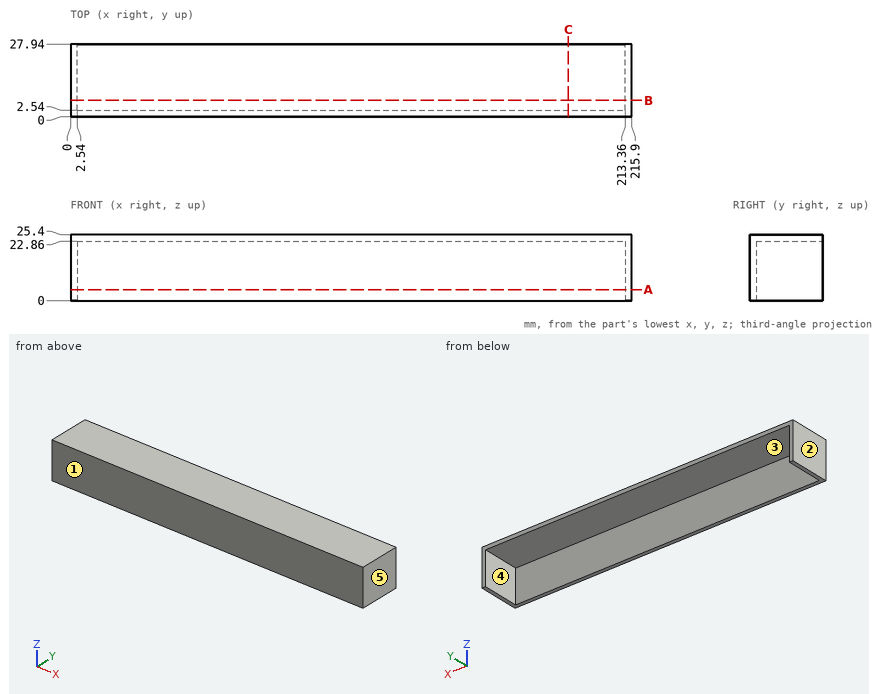
Drawing for the job (mm, zero at the part's lowest x, y, z). A direction names the side the tool comes from. Round coordinates to 2 decimals unless told otherwise and drop trailing zeros. Loops run counter-clockwise (first coordinate to the right, second up) from the corner with the lowest first, then second, coordinate; pieces in that order, holes last. Notation, with made-up numbers: (-11.5, -14.75) -> (44.5, -14.75) arc R13 cw to (44.5, 7.25) -> close; hole circle Ø5 at (-36, 47.25). An arc over 180 degrees is marked (long way). Answer in a Markdown table with one row per item.
Item 1: Saw through at A-A (z = 4.25). Write the cut outline in (x, y), and give its area (3 significant figures).
Answers below:
| item | result |
|---|---|
| outline | (0, 0) -> (215.9, 0) -> (215.9, 27.94) -> (213.36, 27.94) -> (213.36, 2.54) -> (2.54, 2.54) -> (2.54, 27.94) -> (0, 27.94) -> close |
| area | 677 mm² |
Item 2: Which spindle directions (+Z, -Z, +X, -X, +Y, -Y) get a long thin tool onto all of the face, cutting with end or side? Do the marked faces 4 and 5. Say none if no direction does.
Answers below:
| item | result |
|---|---|
| face 4 | -Z, +Y |
| face 5 | +Z, -Z, +X, +Y, -Y |
Item 3: Saw through at C-C (x = 191.5). Write the cut outline in (y, z), and give its area (3 significant figures).
Answers below:
| item | result |
|---|---|
| outline | (0, 0) -> (2.54, 0) -> (2.54, 22.86) -> (27.94, 22.86) -> (27.94, 25.4) -> (0, 25.4) -> close |
| area | 129 mm² |
Item 4: Saw through at B-B (y = 6.25). Write the cut outline in (x, z).
Answers below:
| item | result |
|---|---|
| outline | (0, 0) -> (2.54, 0) -> (2.54, 22.86) -> (213.36, 22.86) -> (213.36, 0) -> (215.9, 0) -> (215.9, 25.4) -> (0, 25.4) -> close |
Item 5: Drill centre lines: L1, parallel to X at y = 25.75, z = 1.25; L2, parallel to Z at x = 39.5, y = 9; L3, parallel to Y at x = 45.5, z = 17.5. Where is each one in solid material? Low to high. Write a range as [from, to].
Answers below:
| item | result |
|---|---|
| L1 | x = [0, 2.54], [213.36, 215.9] |
| L2 | z = [22.86, 25.4] |
| L3 | y = [0, 2.54] |
Item 6: Pin check, flat tips, straight feed: pin 1 (1.5 mm diameter, centred on x = 167.5, y = 11.5, fed in from -Z); pin 2 (5 mm diameter, centred on x = 175.5, z = 5, fed in from +Y). Stop position of each tip, or through.
Answers below:
| item | result |
|---|---|
| pin 1 | stops at z = 22.86 |
| pin 2 | stops at y = 2.54 |
Item 7: Mould opens along X. For the marked faces 1, 2 and 3 say: +X half, -X half, draft (parallel to the pull), parting line (faces both ways), or undercut.
Answers below:
| item | result |
|---|---|
| face 1 | draft |
| face 2 | -X half |
| face 3 | undercut |
